Model file for the job. Use its own axes, mm. Face numbers are marked on the shaded views. A direction names the side the tool comes from. Coordinates: 2 decimals unless noted, no trailing zeros. Order: outer loops, then holes, each group sorted by start corner. A loop starts at its lowest first (then second) coordinate and runs counter-clockwise, first axis right, second up. Notation, with made-up numbers: M 54.5,-33.5 L 63.5,-33.5 A9 cw 63.5,-27.5 Z; hole C 70.5,59 d1. An arc over 180 degrees is marked long. Return JSON: item names as keys, results as strings.
```python
from build123d import *

# Parameters (mm, degrees)
F0_R     = 50.8
F1_DEPTH = 304.8
F2_R     = 5.08
F3_R     = 5.08
F4_R     = 25.4
F5_DEPTH = 101.6
F6_R     = 5.08
F7_R     = 25.4
F8_DEPTH = 101.6
F9_R     = 5.08


with BuildPart() as f1:
    # F0 (on Top) → F1 (new body)
    with BuildSketch(Plane.XY):
        Circle(F0_R)
    extrude(amount=F1_DEPTH)

    # F2
    f2_edges = [f1.edges().sort_by_distance(p)[0] for p in [
        (-50.8, 0, 304.8),
    ]]
    fillet(f2_edges, radius=F2_R)

    # F3
    f3_edges = [f1.edges().sort_by_distance(p)[0] for p in [
        (-50.8, 0, 0),
    ]]
    fillet(f3_edges, radius=F3_R)

    # F4 (on face) → F5 (join)
    with BuildSketch(Plane(origin=(0, 0, 0), x_dir=(1, 0, 0), z_dir=(0, 0, -1))):
        Circle(F4_R)
    extrude(amount=F5_DEPTH)

    # F6
    f6_edges = [f1.edges().sort_by_distance(p)[0] for p in [
        (-25.4, 0, -101.6),
    ]]
    fillet(f6_edges, radius=F6_R)

    # F7 (on face) → F8 (join)
    with BuildSketch(Plane.XY.offset(304.8)):
        Circle(F7_R)
    extrude(amount=F8_DEPTH)

    # F9
    f9_edges = [f1.edges().sort_by_distance(p)[0] for p in [
        (-25.4, 0, 406.4),
    ]]
    fillet(f9_edges, radius=F9_R)


solid = f1.part
```
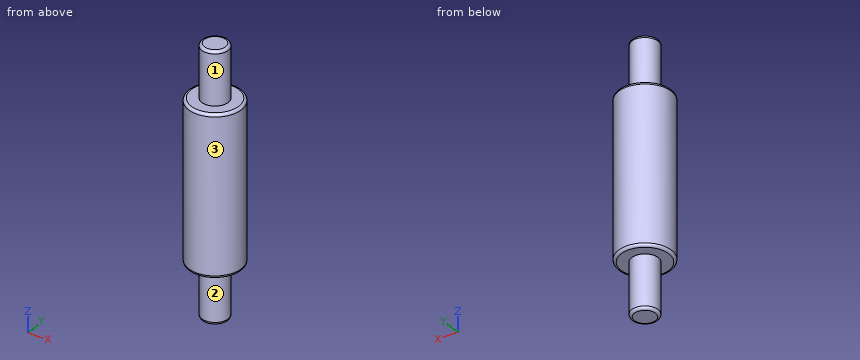
Item 1: Saw through at C-C (z = 242.5). Write the cut outline in (x, y), and give its area (3 significant figures).
Check result:
{"outline": "C 0,0 d101.6", "area": "8,110 mm2"}
Item 2: 3-axis set-ups, long thin cutter, end or side, ignore diameter. For the marked faces 1, 2 and 3: which of +Z, -Z, +X, -X, +Y, -Y reach the whole face in a straight line?
Check result:
{"face 1": "+Z", "face 2": "-Z", "face 3": "+Z, -Z"}
Item 3: Drop flat-ended pins along their axis: pin 1 Ø2 at (y, z) = (-24.5, 245) entering from +X; pin 2 Ø2 at (x, z) = (11.5, 245) entering from -Y; pin 3 Ø12 at (y, z) = (-21, 96.5) entering from +X. Give the stop position or say it passes through.
Check result:
{"pin 1": "stops at x = 45.04", "pin 2": "stops at y = -49.7", "pin 3": "stops at x = 48.53"}
Item 4: Wall check: line 1 (Z direction, x = -28, y = 36.5); line 2 (Y direction, x = -0.5, z = 226.5); line 3 (X direction, y = -33, z = 250). Give the ranges that are in metal, low to high.
Check result:
{"line 1": "z = 0.01 to 304.79", "line 2": "y = -50.8 to 50.8", "line 3": "x = -38.62 to 38.62"}
Item 5: Saw through at A-A (x = 0). Write the cut outline in (y, z).
Check result:
{"outline": "M -50.8,5.08 A5.08 ccw -45.72,0 L -25.4,0 L -25.4,-96.52 A5.08 ccw -20.32,-101.6 L 20.32,-101.6 A5.08 ccw 25.4,-96.52 L 25.4,0 L 45.72,0 A5.08 ccw 50.8,5.08 L 50.8,299.72 A5.08 ccw 45.72,304.8 L 25.4,304.8 L 25.4,401.32 A5.08 ccw 20.32,406.4 L -20.32,406.4 A5.08 ccw -25.4,401.32 L -25.4,304.8 L -45.72,304.8 A5.08 ccw -50.8,299.72 Z"}
